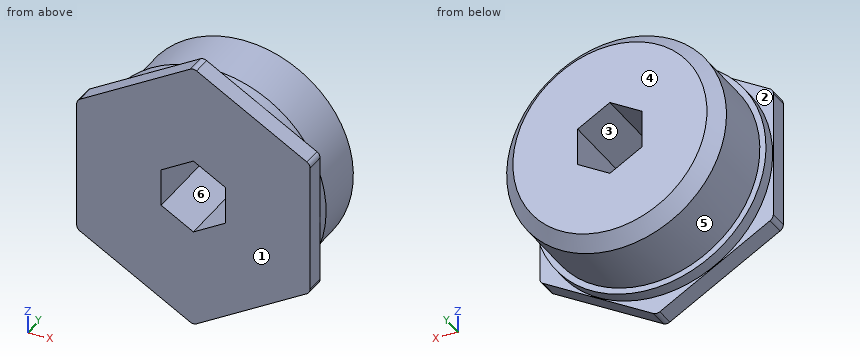
from build123d import *

# Parameters (mm, degrees)
BOSS_EXTRUDE1_DEPTH      = 1.5
FILLET1_R                = 0.5
SKETCH2_R                = 9
BOSS_EXTRUDE2_DEPTH      = 1
SKETCH3_R                = 8.525
BOSS_EXTRUDE3_DEPTH      = 4
BOSS_EXTRUDE4_DEPTH      = 1
BOSS_EXTRUDE4_DEPTH_BACK = 1
SKETCH5_R                = 8.525
SKETCH6_R                = 8.525
BOSS_EXTRUDE5_DEPTH      = 1
CHAMFER2_SIZE            = 1
CUT_EXTRUDE1_DEPTH       = 17.178541022


with BuildPart() as part:
    # Sketch1 → Boss-Extrude1 (new body)
    with BuildSketch(Plane(origin=(0, 31, 0), x_dir=(1, 0, 0), z_dir=(0, 1, 0))):
        Polygon((0, 10.450039872), (-9.05, 5.225019936), (-9.05, -5.225019936), (0, -10.450039872), (9.05, -5.225019936), (9.05, 5.225019936), align=None)
    extrude(amount=BOSS_EXTRUDE1_DEPTH)

    # Fillet1
    fillet1_edges = [part.edges().sort_by_distance(p)[0] for p in [
        (9.05, 31.75, -5.225019936),
        (9.05, 31.75, 5.225019936),
        (0, 31.75, 10.450039872),
        (-9.05, 31.75, 5.225019936),
        (-9.05, 31.75, -5.225019936),
        (0, 31.75, -10.450039872),
    ]]
    fillet(fillet1_edges, radius=FILLET1_R)

    # Sketch2 → Boss-Extrude2 (add)
    with BuildSketch(Plane(origin=(0, 32.5, 0), x_dir=(1, 0, 0), z_dir=(0, 1, 0))):
        with Locations(Location((0, 0, 0), (0, 0, 270))):
            Circle(SKETCH2_R)
    extrude(amount=BOSS_EXTRUDE2_DEPTH)

    # Sketch3 → Boss-Extrude3 (add)
    with BuildSketch(Plane(origin=(0, 33.5, 0), x_dir=(1, 0, 0), z_dir=(0, 1, 0))):
        with Locations(Location((0, 0, 0), (0, 0, 270))):
            Circle(SKETCH3_R)
    extrude(amount=BOSS_EXTRUDE3_DEPTH)

    # Sketch5 → Boss-Extrude4 (add, two sides: drawn at the far end of the back side and taken through both)
    with BuildSketch(Plane(origin=(0, 37.5, 0), x_dir=(1, 0, 0), z_dir=(0, 1, 0)).offset(-BOSS_EXTRUDE4_DEPTH_BACK)):
        with Locations(Location((0, 0, 0), (0, 0, 270))):
            Circle(SKETCH5_R)
    extrude(amount=BOSS_EXTRUDE4_DEPTH + BOSS_EXTRUDE4_DEPTH_BACK)

    # Sketch6 → Boss-Extrude5 (add)
    with BuildSketch(Plane(origin=(0, 38.5, 0), x_dir=(1, 0, 0), z_dir=(0, 1, 0))):
        with Locations(Location((0, 0, 0), (0, 0, 270))):
            Circle(SKETCH6_R)
    extrude(amount=BOSS_EXTRUDE5_DEPTH)

    # Chamfer2
    chamfer2_edges = [part.edges().sort_by_distance(p)[0] for p in [
        (0, 39.5, -8.525),
    ]]
    chamfer(chamfer2_edges, length=CHAMFER2_SIZE)

    # Sketch4 → Cut-Extrude1 (cut, through all)
    with BuildSketch(Plane(origin=(0, 31, 0), x_dir=(1, 0, 0), z_dir=(0, 1, 0))):
        Polygon((0, 2.886751346), (-2.5, 1.443375673), (-2.5, -1.443375673), (0, -2.886751346), (2.5, -1.443375673), (2.5, 1.443375673), align=None)
    extrude(amount=CUT_EXTRUDE1_DEPTH, mode=Mode.SUBTRACT)


solid = part.part
Read the model definition and answer for the solid it produces. Units are mm, in the model's axes. Face numbers are marked on the shaded views. A direction names the side the tool comes from. Coordinates: 2 decimals unless noted, no trailing zeros. Order: outer loops, then holes, each group sorted by start corner. A loop starts at its lowest first (then second) coordinate and runs counter-clockwise, first axis right, second up. Notation, with made-up numbers: M -38,27.5 L -27,27.5 A21 cw -27,39.5 Z; hole C 86,78.25 d11. An arc over 180 degrees is marked long. Put each result on its own line as item: value. Start each with the question number.
Item 1: Section A-A, the plane z = 0 is taken. Determine the outline of the cut face in (x, y) (3 decimals), plus the area to 3 significant figures.
Item 2: The mould has two halves that part along X. Classify the marked faces 4, 5 and 6: +X half, -X half, draft (parallel to the pull), parting line (faces both ways), or undercut.
Item 3: Section B-B, the plane y = 36.25 is taken. Determine the outline of the cut face in (x, z) (3 decimals).
Item 4: Consider probe 1 along Z at (x, y) = (1, 35.5); probe 2 along Z at (x, y) = (-3, 32); probe 3 along X at (y, z) = (36.25, 5.5). Determine where each line is inside the solid, lowest interval first. Write a range as [from, to].
Item 5: For the marked faces 1, 2 and 3, determine the directions among +Z, -Z, +X, -X, +Y, -Y from which every point of the face is accessible in a straight line to the end or side of a thin tool.
Item 6: Given pin 1 Ø1.4 at (y, z) = (33.5, 0) entering from +X; pin 2 Ø2.5 at (y, z) = (34, 0.5) entering from -X; pin 3 Ø1.5 at (y, z) = (38.5, -6.5) entering from -X; pin 4 Ø5 at (x, z) = (7, 7.5) entering from -Y, each flat-ended and moving along its own axis, determine where each tip first touches the part or whether it passes through.
Computed:
1. outline: M -9.05,31 L -2.5,31 L -2.5,39.5 L -7.525,39.5 L -8.525,38.5 L -8.525,33.5 L -9,33.5 L -9,32.5 L -9.05,32.5 Z; M 2.5,31 L 9.05,31 L 9.05,32.5 L 9,32.5 L 9,33.5 L 8.525,33.5 L 8.525,38.5 L 7.525,39.5 L 2.5,39.5 Z
1. area: 104 mm2
2. face 4: draft
2. face 5: parting line
2. face 6: undercut
3. outline: C 0,0 d17.05; hole M -2.5,-1.443 L 0,-2.887 L 2.5,-1.443 L 2.5,1.443 L 0,2.887 L -2.5,1.443 Z
4. probe 1: z = [-8.47, -2.31], [2.31, 8.47]
4. probe 2: z = [-8.72, 8.72]
4. probe 3: x = [-6.51, 6.51]
5. face 1: +Z, -Z, +X, -X, -Y
5. face 2: +Y
5. face 3: +Y, -Y
6. pin 1: stops at x = 9
6. pin 2: stops at x = -9
6. pin 3: stops at x = -6.29
6. pin 4: stops at y = 31
